Source: CAD feature listing. Evaluate the final solid. Frame: model axes, mm. Face numbers are marked on the shaded views. A direction names the side the tool comes from. Round coordinates to 2 decimals unless told otherwise and drop trailing zeros. Order: outer loops, then holes, each group sorted by start corner. A loop starts at its lowest first (then second) coordinate and runs counter-clockwise, first axis right, second up. Notation, with made-up numbers: (13.5, -28.75) -> (36.5, -28.75) arc R14 cw to (36.5, -19.75) -> close; hole circle Ø7 at (25.25, -35.5). An arc over 180 degrees is marked (long way). One line per item, written item: value. Start each with the question number.
1) Mould query, pull axis X, two halves, no side actions, for the marked faces 1, 2 and 3. Classes: pulls with the +X half, pulls with the -X half, needs draft (parallel to the pull), parting line crosses it, or undercut.
2) Section D-D (x = 8.5). Return the cut outline in (y, z), and give its area (3 significant figures).
3) Section B-B (z = 1.2). Return the cut outline in (x, y).
4) Pin query (flat end, axial travel): P1, Ø2, axis at x = 10, z = 3, coming from the +Y side; P2, Ø1.8, axis at x = 7.5, y = 15, coming from the -Z side. Return the tip coordinate at first contact, or that it passes through.
5) Ray query, L1, parallel to Y at x = 8, z = 4.5; L2, parallel to Y at x = 6.5, z = 3.45; L3, parallel to X at y = 5.75, z = 1.45. Return the intervals inside material, ascending.
6) Section A-A (y = 4.75). Return the cut outline in (x, z).
7) Reachability of the marked faces 4 and 5 from +Z, -Z, +X, -X, +Y, -Y: full face, straight path, thin tool, end or side. Return the list, or none.
8) Section C-C (x = 7). Return the cut outline in (y, z).
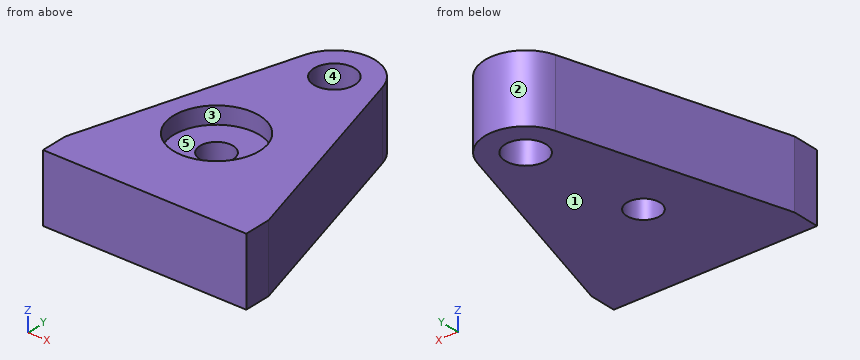
```python
from build123d import *

# Parameters (mm, degrees)
SKETCH1_R                                  = 1.5
BOSS_EXTRUDE1_DEPTH                        = 5
CBORE_FOR_2_HEX_MACHINE_SCREW1_D           = 2.4384
CBORE_FOR_2_HEX_MACHINE_SCREW1_CBORE_D     = 6.35
CBORE_FOR_2_HEX_MACHINE_SCREW1_CBORE_DEPTH = 1.27


with BuildPart() as part:
    # Sketch1 → Boss-Extrude1 (new body)
    with BuildSketch(Plane.XY):
        with BuildLine():
            Line((15, 0), (10.38, 15.84))
            ThreePointArc((10.38, 15.84), (7.5, 18), (4.62, 15.84))
            Line((4.62, 15.84), (0, 0))
            Line((0, 0), (0, -2))
            Line((0, -2), (15, -2))
            Line((15, -2), (15, 0))
        make_face()
        with Locations((7.5, 15)):
            Circle(SKETCH1_R, mode=Mode.SUBTRACT)
    extrude(amount=BOSS_EXTRUDE1_DEPTH)

    # CBORE for #2 Hex Machine Screw1 (through all)
    with Locations(Plane.XY.offset(5)):
        with Locations((6.423403237, 5.750188816)):
            CounterBoreHole(CBORE_FOR_2_HEX_MACHINE_SCREW1_D / 2, CBORE_FOR_2_HEX_MACHINE_SCREW1_CBORE_D / 2, CBORE_FOR_2_HEX_MACHINE_SCREW1_CBORE_DEPTH)


solid = part.part
```
Findings:
1. face 1: needs draft
1. face 2: parting line crosses it
1. face 3: undercut
2. outline: (-2, 0) -> (13.88, 0) -> (13.88, 5) -> (8.15, 5) -> (8.15, 3.73) -> (3.35, 3.73) -> (3.35, 5) -> (-2, 5) -> close; (16.12, 0) -> (17.83, 0) -> (17.83, 5) -> (16.12, 5) -> close
2. area: 81.9 mm2
3. outline: (0, -2) -> (15, -2) -> (15, 0) -> (10.38, 15.84) arc R3 ccw to (4.62, 15.84) -> (0, 0) -> close; hole circle Ø2.44 at (6.42, 5.75); hole circle Ø3 at (7.5, 15)
4. P1: y = 17.6
4. P2: through
5. L1: -2 to 2.99, 8.51 to 13.59, 16.41 to 17.96
5. L2: -2 to 4.53, 6.97 to 13.88, 16.12 to 17.83
5. L3: 1.68 to 5.2, 7.64 to 13.32
6. outline: (1.39, 0) -> (5.73, 0) -> (5.73, 3.73) -> (3.41, 3.73) -> (3.41, 5) -> (1.39, 5) -> close; (7.12, 0) -> (13.61, 0) -> (13.61, 5) -> (9.44, 5) -> (9.44, 3.73) -> (7.12, 3.73) -> close
7. face 4: +Z, -Z
7. face 5: +Z
8. outline: (-2, 0) -> (4.68, 0) -> (4.68, 3.73) -> (2.63, 3.73) -> (2.63, 5) -> (-2, 5) -> close; (6.82, 0) -> (13.59, 0) -> (13.59, 5) -> (8.87, 5) -> (8.87, 3.73) -> (6.82, 3.73) -> close; (16.41, 0) -> (17.96, 0) -> (17.96, 5) -> (16.41, 5) -> close
